For this review, take the finished solid that the model builds, in its own axes (mm). Face numbers are marked on the shaded views. A direction names the side the tool comes from. Round coordinates to 2 decimals unless told otherwise and drop trailing zeros. Order: outer loops, then holes, each group sorted by start corner. A loop starts at its lowest first (then second) coordinate and runs counter-clockwise, first axis right, second up. Notation, with made-up numbers: (-4, 5.25) - (15, 5.25) arc R9 cw to (15, 20.25) - close; hole circle Ø6 at (-39, 13). An arc over 180 degrees is marked (long way). Write each question's results on one line, items separated by ' | '. Start each with the question number.
(1) Take a section at B-B, the plane x = 34.75. Give the boundary of the cut face in (y, z), plus the area to 4 significant figures.
(2) Take a section at A-A, the plane y = 0. Give the boundary of the cut face in (x, z).
(3) Insertion check: pin 1 Ø18.5 at (x, y) = (34.75, 0) entering from +Z; pin 2 Ø5 at (x, y) = (38.462, 18.442) entering from +Z. Each pin has a flat end and moves straight along its axis. Give the tip position at first contact, or say it passes through.
(4) For L1, parallel to X at y = -4, z = 20.75; L2, parallel to Y at x = 24, z = 3.75; L3, parallel to Z at x = 23.5, y = -0.5, list the stretches that pass through material, from the lowest coordinate up. Write a range as from..to.
(5) Take a section at C-C, the plane z = 9.75. Give the boundary of the cut face in (x, y), plus the area to 3 significant figures.
(6) For the marked faces 4 and 5, list the 3-axis set-ups (+Z, -Z, +X, -X, +Y, -Y) from which the entire face can be reached by the end or side of a thin tool; tool diameter is ignored.
(7) Draft analysis for pull direction Y (two halves, no side actions). For the marked faces 1, 2 and 3, state which applies: pulls with the +Y half, pulls with the -Y half, needs draft (parallel to the pull), parting line crosses it, or undercut.
(8) Take a section at D-D, the plane x = 16. Give the boundary of the cut face in (y, z), plus the area to 3 significant figures.
```python
from build123d import *

# Parameters (mm, degrees)
F0_W     = 90
F0_H     = 50
F0_W_2   = 85
F0_H_2   = 45
F1_DEPTH = 3
F2_DEPTH = 26
F3_R     = 2
F4_R     = 5.75
F5_DEPTH = 3
F6_R     = 1.6
F7_DEPTH = 25


with BuildPart() as f1:
    # F0 (on Top) → F1 (new body)
    with BuildSketch(Plane.XY):
        Rectangle(F0_W, F0_H)
        Rectangle(F0_W_2, F0_H_2, mode=Mode.SUBTRACT)
        Rectangle(F0_W_2, F0_H_2)
    extrude(amount=F1_DEPTH)

    # F0 (on Top) → F2 (join)
    with BuildSketch(Plane.XY):
        Rectangle(F0_W, F0_H)
        Rectangle(F0_W_2, F0_H_2, mode=Mode.SUBTRACT)
    extrude(amount=F2_DEPTH)

    # F3
    f3_edges = [f1.edges().sort_by_distance(p)[0] for p in [
        (-45, -25, 13),
        (45, -25, 13),
        (-45, 25, 13),
        (45, 25, 13),
    ]]
    fillet(f3_edges, radius=F3_R)

    # F4 (on face) → F5 (cut, through all)
    with BuildSketch(Plane.XY.offset(3)):
        with Locations((34.75, 0)):
            Circle(F4_R)
    extrude(amount=-F5_DEPTH, mode=Mode.SUBTRACT)

    # F6 (on face) → F7 (cut)
    with BuildSketch(Plane(origin=(0, 0, 0), x_dir=(1, 0, 0), z_dir=(0, 0, -1))):
        with Locations((-38.462, -18.442)):
            Circle(F6_R)
        with Locations((-38.462, 18.442)):
            Circle(F6_R)
        with Locations((38.462, 18.442)):
            Circle(F6_R)
        with Locations((38.462, -18.442)):
            Circle(F6_R)
    extrude(amount=-F7_DEPTH, mode=Mode.SUBTRACT)


solid = f1.part
```
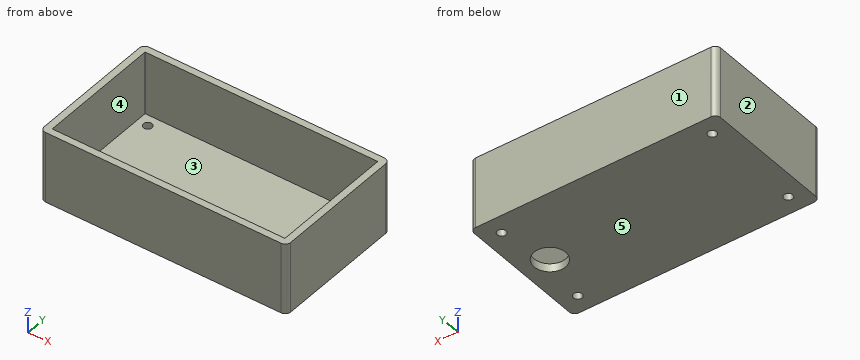
Results below:
1) outline: (-25, 0) - (-5.75, 0) - (-5.75, 3) - (-22.5, 3) - (-22.5, 26) - (-25, 26) - close; (5.75, 0) - (25, 0) - (25, 26) - (22.5, 26) - (22.5, 3) - (5.75, 3) - close | area: 230.5 mm^2
2) outline: (-45, 0) - (29, 0) - (29, 3) - (-42.5, 3) - (-42.5, 26) - (-45, 26) - close; (40.5, 0) - (45, 0) - (45, 26) - (42.5, 26) - (42.5, 3) - (40.5, 3) - close
3) pin 1: stops at z = 26 | pin 2: stops at z = 3
4) L1: x = -45..-42.5, 42.5..45 | L2: y = -25..-22.5, 22.5..25 | L3: z = 0..3
5) outline: (-45, -23) arc R2 ccw to (-43, -25) - (43, -25) arc R2 ccw to (45, -23) - (45, 23) arc R2 ccw to (43, 25) - (-43, 25) arc R2 ccw to (-45, 23) - close; hole (-42.5, -22.5) - (42.5, -22.5) - (42.5, 22.5) - (-42.5, 22.5) - close | area: 672 mm^2
6) face 4: +Z | face 5: -Z, +X, -X, +Y, -Y
7) face 1: pulls with the +Y half | face 2: needs draft | face 3: undercut
8) outline: (-25, 0) - (25, 0) - (25, 26) - (22.5, 26) - (22.5, 3) - (-22.5, 3) - (-22.5, 26) - (-25, 26) - close | area: 265 mm^2
